Geometry: final body of the model. Coordinates: model frame, mm. Face numbers are marked on the shaded views. A direction names the side the tool comes from. Give positions to 0.01 mm unless a question says otherwise; leave off trailing zeros. Write each loop counter-clockwise with the first axis right and the second up, starting at its lowest first coordinate (ties: lowest second). Pieces come first, ordered by that corner, then holes. Notation, with made-up numbers: (76, 5.5) - (120, 5.5) arc R25 ccw to (120, 32.5) - close; hole circle Ø6 at (-32, 54). An arc over 180 degrees is marked (long way). Return JSON: item names as keys, results as strings.
from build123d import *

# Parameters (mm, degrees)
SKETCH1_W             = 15
SKETCH1_H             = 50
BOSS_EXTRUDE1_DEPTH   = 16
SKETCH2_W             = 13
SKETCH2_H             = 8
CUT_EXTRUDE1_DEPTH    = 6
M4_TAPPED_HOLE2_D     = 3.3
M4_TAPPED_HOLE2_DEPTH = 6
M4_TAPPED_HOLE2_TIP   = 0.991420021


with BuildPart() as part:
    # Sketch1 → Boss-Extrude1 (new body)
    with BuildSketch(Plane(origin=(0, 0, 0), x_dir=(1, 0, 0), z_dir=(0, 1, 0))):
        with Locations((7.5, 25)):
            Rectangle(SKETCH1_W, SKETCH1_H)
    extrude(amount=BOSS_EXTRUDE1_DEPTH)

    # Sketch2 → Cut-Extrude1 (cut)
    with BuildSketch(Plane(origin=(0, 16, 0), x_dir=(1, 0, 0), z_dir=(0, 1, 0))):
        with Locations((8.5, 5.5)):
            Rectangle(SKETCH2_W, SKETCH2_H)
        with Locations((8.5, 15.3)):
            Rectangle(SKETCH2_W, SKETCH2_H)
        with Locations((8.5, 25.1)):
            Rectangle(SKETCH2_W, SKETCH2_H)
        with Locations((8.5, 34.9)):
            Rectangle(SKETCH2_W, SKETCH2_H)
        with Locations((8.5, 44.7)):
            Rectangle(SKETCH2_W, SKETCH2_H)
    extrude(amount=-CUT_EXTRUDE1_DEPTH, mode=Mode.SUBTRACT)

    # M4 Tapped Hole2
    with Locations(Plane(origin=(0, 10, 0), x_dir=(1, 0, 0), z_dir=(0, 1, 0))):
        with Locations((9, 5.5), (9, 15.3), (9, 25.1), (9, 34.9), (9, 44.7)):
            Hole(M4_TAPPED_HOLE2_D / 2, depth=M4_TAPPED_HOLE2_DEPTH)
            with Locations((0, 0, -(M4_TAPPED_HOLE2_DEPTH + M4_TAPPED_HOLE2_TIP / 2))):  # 118° drill point
                Cone(0, M4_TAPPED_HOLE2_D / 2, M4_TAPPED_HOLE2_TIP, mode=Mode.SUBTRACT)


solid = part.part
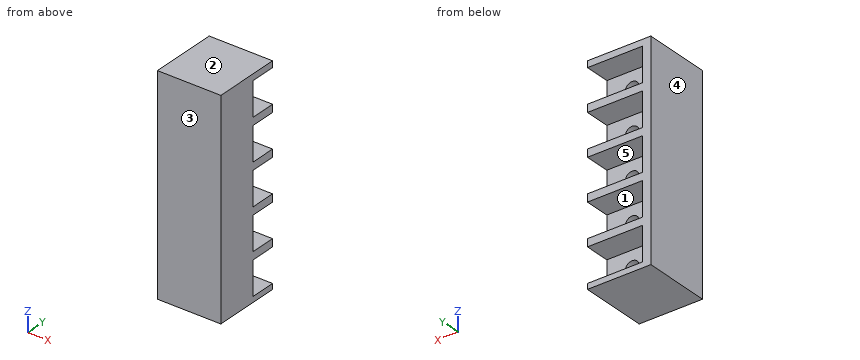
Q1. Mould query, pull axis Z, two halves, no side actions, for the marked faces 1, 2 and 3. Classes: pulls with the +Z half, pulls with the -Z half, needs draft (parallel to the pull), parting line crosses it, or undercut.
Answer key:
{"face 1": "undercut", "face 2": "pulls with the +Z half", "face 3": "needs draft"}
Q2. Section query B-B, the plane y = 7.75. Return the cut outline in (x, z), plus the area to 3 significant figures.
Answer key:
{"outline": "(0, -50) - (15, -50) - (15, 0) - (0, 0) - close; hole circle Ø3.3 at (9, -44.7); hole circle Ø3.3 at (9, -34.9); hole circle Ø3.3 at (9, -25.1); hole circle Ø3.3 at (9, -15.3); hole circle Ø3.3 at (9, -5.5)", "area": "707 mm^2"}
Q3. Section query A-A, the plane x = 3. Return the cut outline in (y, z), plus the area to 3 significant figures.
Answer key:
{"outline": "(0, -50) - (16, -50) - (16, -48.7) - (10, -48.7) - (10, -40.7) - (16, -40.7) - (16, -38.9) - (10, -38.9) - (10, -30.9) - (16, -30.9) - (16, -29.1) - (10, -29.1) - (10, -21.1) - (16, -21.1) - (16, -19.3) - (10, -19.3) - (10, -11.3) - (16, -11.3) - (16, -9.5) - (10, -9.5) - (10, -1.5) - (16, -1.5) - (16, 0) - (0, 0) - close", "area": "560 mm^2"}
Q4. Section query C-C, the plane z = -38. Return the cut outline in (x, y), plus the area to 3 significant figures.
Answer key:
{"outline": "(0, 0) - (15, 0) - (15, 10) - (2, 10) - (2, 16) - (0, 16) - close", "area": "162 mm^2"}
Q5. Set-up query: the marked faces 4 and 5. Return all of +Z, -Z, +X, -X, +Y, -Y with unobstructed straight access to the full face (end or side cutting, diameter ignored); none if empty.
Answer key:
{"face 4": "+Z, -Z, -X, +Y, -Y", "face 5": "+X, +Y"}
Q6. Material intervals for probe 1 along Z at (x, y) = (14, 13); probe 2 along Z at (x, y) = (9, 6.15); probe 3 along X at (y, z) = (8.85, -44.7), sorted ascending. Write a range as [from, to].
Answer key:
{"probe 1": "z = [-50, -48.7], [-40.7, -38.9], [-30.9, -29.1], [-21.1, -19.3], [-11.3, -9.5], [-1.5, 0]", "probe 2": "z = [-50, -46.35], [-43.05, -36.55], [-33.25, -26.75], [-23.45, -16.95], [-13.65, -7.15], [-3.85, 0]", "probe 3": "x = [0, 7.35], [10.65, 15]"}
Q7. Pin query (flat end, axial travel): P1, Ø5.5, axis at x = 9, z = -34.9, coming from the +Y side; P2, Ø1.8, axis at y = 12.5, z = -14.5, coming from the +X side. Return the tip coordinate at first contact, or that it passes through.
Answer key:
{"P1": "stops at y = 10", "P2": "stops at x = 2"}
